The model under review builds one solid part; all positions refer to its coordinate system, in mm. Give positions to 0.01 mm unless a question says otherwise; leave off trailing zeros. Order: outer loops, then holes, each group sorted by start corner. A loop starts at its lowest first (then second) coordinate and runs counter-clockwise, first axis right, second up. Notation, with made-up numbers: (4.5, -9) -> (56.5, -9) arc R36 ccw to (56.5, 25) -> close; hole circle Ø9 at (39, -38.75). An arc over 180 degrees is marked (long way). Use one line per item in the form item = value.
```python
from build123d import *

# Parameters (mm, degrees)
SKETCH1_R           = 1.5875
BOSS_EXTRUDE1_DEPTH = 1.5875
CUT_EXTRUDE1_DEPTH  = 10


with BuildPart() as part:
    # Sketch1 → Boss-Extrude1 (new body)
    with BuildSketch(Plane.XZ.offset(-9.652)):
        with BuildLine():
            Line((-9.649529152, -57.088970848), (-9.649529152, -56.4515))
            ThreePointArc((-9.649529152, -56.4515), (0, -46.801970848), (9.649529152, -56.4515))
            Line((9.649529152, -56.4515), (9.649529152, -57.088970848))
            ThreePointArc((9.649529152, -57.088970848), (10.579465122, -59.334034878), (12.824529152, -60.263970848))
            Line((12.824529152, -60.263970848), (83.228304068, -60.263970848))
            ThreePointArc((83.228304068, -60.263970848), (85.473368098, -59.334034878), (86.403304068, -57.088970848))
            Line((86.403304068, -57.088970848), (86.403304068, -53.197827078))
            ThreePointArc((86.403304068, -53.197827078), (89.303980599, -46.194974456), (96.306833221, -43.294297925))
            Line((96.306833221, -43.294297925), (97.90475189, -43.294297925))
            ThreePointArc((97.90475189, -43.294297925), (98.735652203, -42.90897515), (99.641972868, -42.776869801))
            Line((99.641972868, -42.776869801), (103.212691826, -42.776869801))
            ThreePointArc((103.212691826, -42.776869801), (104.267987777, -41.630083879), (104.650470848, -40.119297925))
            Line((104.650470848, -40.119297925), (104.650470848, 40.119297925))
            ThreePointArc((104.650470848, 40.119297925), (104.267987777, 41.630083879), (103.212691826, 42.776869801))
            Line((103.212691826, 42.776869801), (99.641972868, 42.776869801))
            ThreePointArc((99.641972868, 42.776869801), (98.735652203, 42.90897515), (97.90475189, 43.294297925))
            Line((97.90475189, 43.294297925), (96.306833221, 43.294297925))
            ThreePointArc((96.306833221, 43.294297925), (89.303980599, 46.194974456), (86.403304068, 53.197827078))
            Line((86.403304068, 53.197827078), (86.403304068, 57.088970848))
            ThreePointArc((86.403304068, 57.088970848), (85.473368098, 59.334034878), (83.228304068, 60.263970848))
            Line((83.228304068, 60.263970848), (12.824529152, 60.263970848))
            ThreePointArc((12.824529152, 60.263970848), (10.579465122, 59.334034878), (9.649529152, 57.088970848))
            Line((9.649529152, 57.088970848), (9.649529152, 56.4515))
            ThreePointArc((9.649529152, 56.4515), (0, 46.801970848), (-9.649529152, 56.4515))
            Line((-9.649529152, 56.4515), (-9.649529152, 57.088970848))
            ThreePointArc((-9.649529152, 57.088970848), (-10.579465122, 59.334034878), (-12.824529152, 60.263970848))
            Line((-12.824529152, 60.263970848), (-83.228304068, 60.263970848))
            ThreePointArc((-83.228304068, 60.263970848), (-85.473368098, 59.334034878), (-86.403304068, 57.088970848))
            Line((-86.403304068, 57.088970848), (-86.403304068, 53.197827078))
            ThreePointArc((-86.403304068, 53.197827078), (-89.303980599, 46.194974456), (-96.306833221, 43.294297925))
            Line((-96.306833221, 43.294297925), (-101.475470848, 43.294297925))
            ThreePointArc((-101.475470848, 43.294297925), (-103.720534878, 42.364361955), (-104.650470848, 40.119297925))
            Line((-104.650470848, 40.119297925), (-104.650470848, -40.119297925))
            ThreePointArc((-104.650470848, -40.119297925), (-103.720534878, -42.364361955), (-101.475470848, -43.294297925))
            Line((-101.475470848, -43.294297925), (-96.306833221, -43.294297925))
            ThreePointArc((-96.306833221, -43.294297925), (-89.303980599, -46.194974456), (-86.403304068, -53.197827078))
            Line((-86.403304068, -53.197827078), (-86.403304068, -57.088970848))
            ThreePointArc((-86.403304068, -57.088970848), (-85.473368098, -59.334034878), (-83.228304068, -60.263970848))
            Line((-83.228304068, -60.263970848), (-12.824529152, -60.263970848))
            ThreePointArc((-12.824529152, -60.263970848), (-10.579465122, -59.334034878), (-9.649529152, -57.088970848))
        make_face()
        with Locations(Location((18.12925, 51.53025, 0), (0, 0, 90))):
            Circle(SKETCH1_R, mode=Mode.SUBTRACT)
        with Locations(Location((18.12925, -51.53025, 0), (0, 0, 90))):
            Circle(SKETCH1_R, mode=Mode.SUBTRACT)
        with Locations(Location((95.91675, -35.65525, 0), (0, 0, 90))):
            Circle(SKETCH1_R, mode=Mode.SUBTRACT)
        with Locations(Location((78.45425, 51.53025, 0), (0, 0, 90))):
            Circle(SKETCH1_R, mode=Mode.SUBTRACT)
        with Locations(Location((-95.91675, 35.65525, 0), (0, 0, 90))):
            Circle(SKETCH1_R, mode=Mode.SUBTRACT)
        with Locations(Location((-78.45425, -51.53025, 0), (0, 0, 90))):
            Circle(SKETCH1_R, mode=Mode.SUBTRACT)
        with Locations(Location((-18.12925, -51.53025, 0), (0, 0, 90))):
            Circle(SKETCH1_R, mode=Mode.SUBTRACT)
        with Locations(Location((-95.91675, -35.65525, 0), (0, 0, 90))):
            Circle(SKETCH1_R, mode=Mode.SUBTRACT)
        with Locations(Location((-78.45425, 51.53025, 0), (0, 0, 90))):
            Circle(SKETCH1_R, mode=Mode.SUBTRACT)
        with Locations(Location((95.91675, 35.65525, 0), (0, 0, 90))):
            Circle(SKETCH1_R, mode=Mode.SUBTRACT)
        with Locations(Location((78.45425, -51.53025, 0), (0, 0, 90))):
            Circle(SKETCH1_R, mode=Mode.SUBTRACT)
        with Locations(Location((-18.12925, 51.53025, 0), (0, 0, 90))):
            Circle(SKETCH1_R, mode=Mode.SUBTRACT)
    extrude(amount=-BOSS_EXTRUDE1_DEPTH)

    # Sketch2 → Cut-Extrude1 (cut)
    with BuildSketch(Plane(origin=(0, 11.2395, 0), x_dir=(1, 0, 0), z_dir=(0, 1, 0))):
        with BuildLine():
            ThreePointArc((-38.445, 27), (-42.132350647, 28.527350647), (-40.605, 24.84))
            Line((-40.605, 24.84), (-40.605, 27))
            Line((-40.605, 27), (-38.445, 27))
        make_face()
        with BuildLine():
            Line((-40.605, 27), (-40.605, 24.84))
            ThreePointArc((-40.605, 24.84), (-39.077649353, 25.472649353), (-38.445, 27))
            Line((-38.445, 27), (-40.605, 27))
        make_face()
        with BuildLine():
            Line((-38.445, -33), (-40.605, -33))
            Line((-40.605, -33), (-40.605, -30.84))
            ThreePointArc((-40.605, -30.84), (-42.132350647, -34.527350647), (-38.445, -33))
        make_face()
        with BuildLine():
            Line((-40.605, -30.84), (-40.605, -33))
            Line((-40.605, -33), (-38.445, -33))
            ThreePointArc((-38.445, -33), (-39.077649353, -31.472649353), (-40.605, -30.84))
        make_face()
        with BuildLine():
            ThreePointArc((40.605, -30.84), (39.077649353, -31.472649353), (38.445, -33))
            Line((38.445, -33), (40.605, -33))
            Line((40.605, -33), (40.605, -30.84))
        make_face()
        with BuildLine():
            Line((40.605, -33), (38.445, -33))
            ThreePointArc((38.445, -33), (40.605, -35.16), (42.765, -33))
            ThreePointArc((42.765, -33), (42.132350647, -31.472649353), (40.605, -30.84))
            Line((40.605, -30.84), (40.605, -33))
        make_face()
        with BuildLine():
            ThreePointArc((42.765, 27), (40.605, 29.16), (38.445, 27))
            Line((38.445, 27), (40.605, 27))
            Line((40.605, 27), (40.605, 24.84))
            ThreePointArc((40.605, 24.84), (42.132350647, 25.472649353), (42.765, 27))
        make_face()
        with BuildLine():
            Line((40.605, 27), (38.445, 27))
            ThreePointArc((38.445, 27), (39.077649353, 25.472649353), (40.605, 24.84))
            Line((40.605, 24.84), (40.605, 27))
        make_face()
    extrude(amount=-CUT_EXTRUDE1_DEPTH, mode=Mode.SUBTRACT)


solid = part.part
```
1. Add section B-B on y = 10.75. Count the separate pieces of the cut face and the enclosed holes in it, then the cut area to 3 significant figures.
Values:
separate_pieces = 1
enclosed_holes = 16
area = 23,400 mm^2
2. For L1, parallel to X at y = 10.75, z = -27 (3 decimals); L2, parallel to Z at x = 39.5, y = 10.4; L3, parallel to Z at x = -94.5, y = 10.2, list the stretches that pass through material, from the lowest coordinate up.
Values:
L1 = -104.65 to -42.765, -38.445 to 38.445, 42.765 to 104.65
L2 = -60.26 to -28.86, -25.14 to 31.14, 34.86 to 60.26
L3 = -43.46 to -36.37, -34.94 to 34.94, 36.37 to 43.46
3. For pin 1 Ø4 at (x, z) = (-40.605, -27) entering from +Y; pin 2 Ø0.5 at (y, z) = (11, 55) entering from +X; pin 3 Ø0.8 at (x, y) = (97, 10.5) entering from +Z, all flat-tipped, find the tip position at first contact; note any pin that passes through.
Values:
pin_1 = through
pin_2 = 86.4
pin_3 = 43.29
4. Add section A-A on x = 0. Give the boundary of the cut face in (y, z), then the cut area to 3 significant figures.
Values:
outline = (9.65, -46.8) -> (11.24, -46.8) -> (11.24, 46.8) -> (9.65, 46.8) -> close
area = 149 mm^2
5. The part is to be moulded in two halves that separate along X. For faces 1 (the face through (0.212, 10.435, 46.804)), 2 (the face through (-89.2, 10.4, 46.3)), 3 (the face through (-1, 9.652, 1)), say which applies: +X half, -X half, draft (parallel to the pull), parting line (faces both ways), or undercut.
Values:
face_1 = undercut
face_2 = -X half
face_3 = draft
